```python
from build123d import *

# Parameters (mm, degrees)
SKETCH_1_W         = 35.99999999
SKETCH_1_H         = 13
SKETCH_1_R         = 2.999999999
SKETCH_1_R_2       = 0.8
SKETCH_1_R_3       = 1.500000001
SKETCH_1_R_4       = 0.799999999
SKETCH_1_R_5       = 0.799999997
SKETCH_1_R_6       = 0.799999998
SKETCH_1_R_7       = 2.999999997
EXTRUDE_1_DEPTH    = 1.5
SKETCH_2_W         = 5
SKETCH_2_H         = 3
SKETCH_2_W_2       = 4.999999998
EXTRUDE_2_DEPTH    = 8.5
HOLE_WIZARD_M2_1_D = 1.6


with BuildPart() as part:
    # 스케치1 → 돌출1 (new body)
    with BuildSketch(Plane.XY):
        with Locations((-1e-09, -2.4)):
            Rectangle(SKETCH_1_W, SKETCH_1_H)
        with Locations((-10.205880656, -2.000000001)):
            Circle(SKETCH_1_R, mode=Mode.SUBTRACT)
        with Locations((-14.536007677, 0.5)):
            Circle(SKETCH_1_R_2, mode=Mode.SUBTRACT)
        with Locations((-5.875753638, 0.499999998)):
            Circle(SKETCH_1_R_2, mode=Mode.SUBTRACT)
        with Locations((-1e-09, 0)):
            Circle(SKETCH_1_R_3, mode=Mode.SUBTRACT)
        with Locations((-10.205880656, -7.000000001)):
            Circle(SKETCH_1_R_4, mode=Mode.SUBTRACT)
        with Locations(Location((10.205880654, -7.000000001, 0), (0, 0, 180))):
            Circle(SKETCH_1_R_5, mode=Mode.SUBTRACT)
        with Locations(Location((5.875753636, 0.499999998, 0), (0, 0, 180))):
            Circle(SKETCH_1_R_5, mode=Mode.SUBTRACT)
        with Locations(Location((14.536007674, 0.5, 0), (0, 0, 180))):
            Circle(SKETCH_1_R_6, mode=Mode.SUBTRACT)
        with Locations(Location((10.205880654, -2.000000001, 0), (0, 0, 180))):
            Circle(SKETCH_1_R_7, mode=Mode.SUBTRACT)
    extrude(amount=EXTRUDE_1_DEPTH)

    # 스케치2 → 돌출2 (add)
    with BuildSketch(Plane.XY.offset(1.5)):
        with Locations((-15.499999996, -7.4)):
            Rectangle(SKETCH_2_W, SKETCH_2_H)
        with Locations((15.499999995, -7.4)):
            Rectangle(SKETCH_2_W_2, SKETCH_2_H)
    extrude(amount=EXTRUDE_2_DEPTH)

    # M2 탭을 위한 탭 드릴1 (through all)
    with Locations(Plane(origin=(-15.499999996, -8.9, 5), x_dir=(-1, 0, 0), z_dir=(0, -1, 0))):
        with Locations((0, 0), (-30.999999991, 0)):
            Hole(HOLE_WIZARD_M2_1_D / 2)


solid = part.part
```
Build history of the part. All positions in model axes, mm. A direction names the side the tool comes from. Round coordinates to 2 decimals unless told otherwise and drop trailing zeros. Order: outer loops, then holes, each group sorted by start corner. A loop starts at its lowest first (then second) coordinate and runs counter-clockwise, first axis right, second up. Notation, with made-up numbers: (65, 74) - (105, 74) arc R38 cw to (105, 113) - close; hole circle Ø10 at (-16, 0.25). An arc over 180 degrees is marked (long way). Use a Markdown table: item, result.
1) Saw through at D-D on y = -3.5. Write the cut outline in (x, z).
Recorded:
| item | result |
|---|---|
| outline | (-18, 0) - (-12.8, 0) - (-12.8, 1.5) - (-18, 1.5) - close; (-7.61, 0) - (7.61, 0) - (7.61, 1.5) - (-7.61, 1.5) - close; (12.8, 0) - (18, 0) - (18, 1.5) - (12.8, 1.5) - close |
2) Saw through at B-B on z = 2.5. Write the cut outline in (x, y), and give its area (3 significant figures).
Recorded:
| item | result |
|---|---|
| outline | (-18, -8.9) - (-13, -8.9) - (-13, -5.9) - (-18, -5.9) - close; (13, -8.9) - (18, -8.9) - (18, -5.9) - (13, -5.9) - close |
| area | 30.0 mm² |
3) Pull direction Y, two halves, no side cores. Call faces 1 (the face through (11.005, -7.035, 0.74)), 2 (the face through (16, -5.9, 6)), 3 (the face through (0, -2, 0)): pulls with the +Y half, pulls with the -Y half, needs draft (parallel to the pull), parting line crosses it, or undercut.
Recorded:
| item | result |
|---|---|
| face 1 | undercut |
| face 2 | pulls with the +Y half |
| face 3 | needs draft |
4) Wall check: L1, parallel to X at y = -6.85, z = 5; L2, parallel to Y at x = 0, z = 0.4; L3, parallel to Z at x = -10, y = -8. Give the ranges that are in metal, low to high.
Recorded:
| item | result |
|---|---|
| L1 | x = -18 to -16.3, -14.7 to -13, 13 to 14.7, 16.3 to 18 |
| L2 | y = -8.9 to -1.5, 1.5 to 4.1 |
| L3 | z = 0 to 1.5 |
5) Saw through at C-C on x = 0. Write the cut outline in (y, z).
Recorded:
| item | result |
|---|---|
| outline | (-8.9, 0) - (-1.5, 0) - (-1.5, 1.5) - (-8.9, 1.5) - close; (1.5, 0) - (4.1, 0) - (4.1, 1.5) - (1.5, 1.5) - close |
6) Saw through at A-A on y = -7. Write the cut outline in (x, z), and give its area (3 significant figures).
Recorded:
| item | result |
|---|---|
| outline | (-18, 0) - (-11.01, 0) - (-11.01, 1.5) - (-13, 1.5) - (-13, 10) - (-18, 10) - close; (-9.41, 0) - (9.41, 0) - (9.41, 1.5) - (-9.41, 1.5) - close; (11.01, 0) - (18, 0) - (18, 10) - (13, 10) - (13, 1.5) - (11.01, 1.5) - close; hole circle Ø1.6 at (-15.5, 5); hole circle Ø1.6 at (15.5, 5) |
| area | 130 mm² |
7) Tool access for faces 4 (the face through (15, -7, 10)), 5 (the face through (0, -2, 1.5)), 6 (the face through (-13, -7, 6)): list every direction of +Z, -Z, +X, -X, +Y, -Y with a clear straight run to the whole face (end or side of a thin tool).
Recorded:
| item | result |
|---|---|
| face 4 | +Z, +X, -X, +Y, -Y |
| face 5 | +Z, +Y |
| face 6 | +Z, +Y, -Y |
8) Flat gauge pins, fed straight in: pin 1 Ø5 at (x, y) = (-7, -5.5) entering from +Z; pin 2 Ø1.5 at (x, z) = (15.5, 5.5) entering from +Y. Where does each tip first touch, or does it go through?
Recorded:
| item | result |
|---|---|
| pin 1 | stops at z = 1.5 |
| pin 2 | stops at y = -5.9 |
